```python
from build123d import *

# Parameters (mm, degrees)
SKETCH1_R               = 44.45
SKETCH1_R_2             = 38.1
BOSS_EXTRUDE1_DEPTH     = 35.56
CHAMFER1_SIZE           = 7.62
CHAMFER1_SIZE2          = 4.399409051
CUT_EXTRUDE1_DEPTH      = 73.222701417
CUT_EXTRUDE1_DEPTH_BACK = 73.222701417
SKETCH2_R               = 2.54


with BuildPart() as part:
    # Sketch1 → Boss-Extrude1 (new body)
    with BuildSketch(Plane.XY):
        Circle(SKETCH1_R)
        Circle(SKETCH1_R_2, mode=Mode.SUBTRACT)
    extrude(amount=BOSS_EXTRUDE1_DEPTH)

    # Chamfer1
    chamfer1_edges = [part.edges().sort_by_distance(p)[0] for p in [
        (-44.45, 0, 35.56),
    ]]
    chamfer1_side = [part.faces().sort_by_distance(p)[0] for p in [
        (-44.45, 0, 17.78),
    ]]
    chamfer(chamfer1_edges, length=CHAMFER1_SIZE, length2=CHAMFER1_SIZE2, reference=chamfer1_side[0])

    # Sketch2 → Cut-Extrude1 (cut, two sides: drawn at the far end of the back side and taken through both)
    with BuildSketch(Plane(origin=(0, 0, 0), x_dir=(0, 0, -1), z_dir=(1, 0, 0)).offset(-CUT_EXTRUDE1_DEPTH_BACK)):
        with Locations((-16.0782, 0)):
            Circle(SKETCH2_R)
    extrude(amount=CUT_EXTRUDE1_DEPTH + CUT_EXTRUDE1_DEPTH_BACK, mode=Mode.SUBTRACT)


solid = part.part
```
Read the model definition and answer for the solid it produces. Units are mm, in the model's axes. Give positions to 0.01 mm unless a question says otherwise; leave off trailing zeros. Loops run counter-clockwise (first coordinate to the right, second up) from the corner with the lowest first, then second, coordinate; pieces in that order, holes last.
Item 1: Find the intervals of material crossed by line 1 along Y through (x, z) = (0, 24); line 2 along Y through (x, z) = (35, 25), in increasing order.
Item 2: The part is cut by section C-C (z = 15). Write down the section's boundary in (x, y).
Item 3: The part is cut by section A-A (x = 0). Write down the section's boundary in (y, z).
Item 4: The mould has two halves that part along Y. Classify faces 1 (the cylindrical face through (-41.278, 0.763, 13.655)), 2 (the flat face through (14.6, -35.4, 35.56)), 3 (the conical face through (-8.728, -39.307, 35.19)): released by +Y, released by -Y, zero draft, split by the parting line, or undercut.
Item 5: The part is cut by section D-D (z = 7.5). Write down the section's boundary in (x, y).
Item 6: Each of these flat-tipped pins is pushed along its axis until it touches: pin 1 Ø8 at (x, z) = (31.5, 11.5) entering from +Y; pin 2 Ø8 at (y, z) = (-23.5, 22) entering from -X; pin 3 Ø6 at (x, z) = (2, 26) entering from -Y. Where does it stop, or does it pass through?
Item 7: The part is cut by section B-B (y = 0). Write down the section's boundary in (x, z), and give its area (3 significant figures).
Taken from the geometry:
1. line 1: y = -44.45 to -38.1, 38.1 to 44.45
1. line 2: y = -27.4 to -15.05, 15.05 to 27.4
2. outline: (-44.39, -2.3) arc R44.45 ccw to (44.39, -2.3) - (38.03, -2.3) arc R38.1 cw to (-38.03, -2.3) - close; (-44.39, 2.3) - (-38.03, 2.3) arc R38.1 cw to (38.03, 2.3) - (44.39, 2.3) arc R44.45 ccw to start
3. outline: (-44.45, 0) - (-38.1, 0) - (-38.1, 35.56) - (-40.05, 35.56) - (-44.45, 27.94) - close; (38.1, 0) - (44.45, 0) - (44.45, 27.94) - (40.05, 35.56) - (38.1, 35.56) - close
4. face 1: undercut
4. face 2: zero draft
4. face 3: split by the parting line
5. outline: circle Ø88.9 at (0, 0); hole circle Ø76.2 at (0, 0)
6. pin 1: stops at y = 34.92
6. pin 2: stops at x = -39.94
6. pin 3: stops at y = -44.45
7. outline: (-44.45, 0) - (-38.1, 0) - (-38.1, 13.54) - (-44.45, 13.54) - close; (-44.45, 18.62) - (-38.1, 18.62) - (-38.1, 35.56) - (-40.05, 35.56) - (-44.45, 27.94) - close; (38.1, 0) - (44.45, 0) - (44.45, 13.54) - (38.1, 13.54) - close; (38.1, 18.62) - (44.45, 18.62) - (44.45, 27.94) - (40.05, 35.56) - (38.1, 35.56) - close
7. area: 354 mm2
